Input: part model. Units: mm. Frame: model coordinates. Face numbers are marked on the shaded views. A direction names the side the tool comes from. Coordinates: 2 decimals unless noted, no trailing zeros. Loops run counter-clockwise (first coordinate to the right, second up) from the corner with the lowest first, then second, coordinate; pieces in that order, holes last. Notation, with made-up numbers: (-19.5, -6) - (25.5, -6) arc R17 cw to (25.5, 24) - close; hole circle Ø10 at (45, 54.5). An arc over 180 degrees is marked (long way). Use a Markdown table: item, result. Add a question column.
1. Contact query for a flat-ended pin moving along its axis: P1, Ø4, axis at y = -34, z = 23.5, coming from the -X side. Output: stop coordinate, or through.
2. Section query B-B on y = -24. Return the cut outline in (x, z), then the cut area to 3 significant figures.
3. Section query C-C on x = 8. Return the cut outline in (y, z).
4. Access query for the marked faces 1 and 2. Directions: +Z, -Z, +X, -X, +Y, -Y. A direction counts if a zero-diameter tool reaches every point of the face in a straight line with its end or side. Return the directions, or none.
5. Ray query, L1, parallel to Y at x = 38, z = 14.5; L2, parallel to Z at x = 45, y = 25.5; L3, parallel to X at y = 21.5, z = 6.5. Return the intervals inside material, ascending. Write a range as [from, to].
6. Section query A-A on z = -6. Return the cut outline in (x, y).
7. Draft query along Z for the marked faces 3, 4, 5 and 6. Return one class per face: released by +Z, released by -Z, zero draft, split by the parting line, or undercut.
```python
from build123d import *

# Parameters (mm, degrees)
F0_W     = 88.9
F0_H     = 63.5
F1_DEPTH = 55.88
F2_W     = 83.951384
F2_H     = 57.938274
F3_DEPTH = 54.102


with BuildPart() as f1:
    # F0 (on Right) → F1 (new body)
    with BuildSketch(Plane.YZ):
        Rectangle(F0_W, F0_H)
    extrude(amount=F1_DEPTH)

    # F2 (on face) → F3 (cut)
    with BuildSketch(Plane(origin=(0, 0, 0), x_dir=(0, -1, 0), z_dir=(-1, 0, 0))):
        Rectangle(F2_W, F2_H)
    extrude(amount=-F3_DEPTH, mode=Mode.SUBTRACT)


solid = f1.part
```
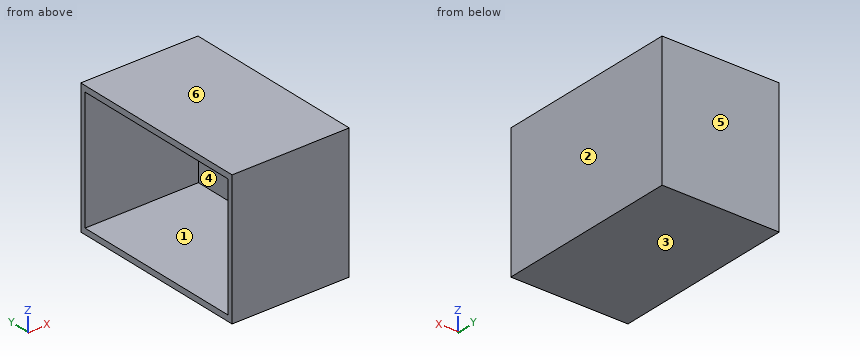
Resolved:
| question | item | result |
|---|---|---|
| 1 | P1 | x = 54.1 |
| 2 | outline | (0, -31.75) - (55.88, -31.75) - (55.88, 31.75) - (0, 31.75) - (0, 28.97) - (54.1, 28.97) - (54.1, -28.97) - (0, -28.97) - close |
| 2 | area | 414 mm² |
| 3 | outline | (-44.45, -31.75) - (44.45, -31.75) - (44.45, 31.75) - (-44.45, 31.75) - close; hole (-41.98, -28.97) - (41.98, -28.97) - (41.98, 28.97) - (-41.98, 28.97) - close |
| 4 | face 1 | -X |
| 4 | face 2 | +Z, -Z, +X, +Y, -Y |
| 5 | L1 | [-44.45, -41.98], [41.98, 44.45] |
| 5 | L2 | [-31.75, -28.97], [28.97, 31.75] |
| 5 | L3 | [54.1, 55.88] |
| 6 | outline | (0, -44.45) - (55.88, -44.45) - (55.88, 44.45) - (0, 44.45) - (0, 41.98) - (54.1, 41.98) - (54.1, -41.98) - (0, -41.98) - close |
| 7 | face 3 | released by -Z |
| 7 | face 4 | undercut |
| 7 | face 5 | zero draft |
| 7 | face 6 | released by +Z |
